Could you check a few things on this model? Use its own coordinates, in mm. A direction names the side the tool comes from. Coordinates: 2 decimals unless noted, no trailing zeros. Write each loop counter-clockwise with the first axis right and the second up, starting at its lowest first coordinate (ties: lowest second). Pieces come first, ordered by that corner, then holes.
Autodesk Inventor part; units mm, degrees
ref_plane "YZ Plane" through (0, 0, 0) normal (1, 0, 0) x (0, 1, 0)
ref_plane "XZ Plane" through (0, 0, 0) normal (0, 1, 0) x (-1, 0, 0)
ref_plane "XY Plane" through (0, 0, 0) normal (0, 0, 1) x (1, 0, 0)
sketch "Sketch1" plane through (0, 0, 0) normal (1, 0, 0) x (0, 1, 0)
  line L0 (0, 0) -> (50.8, 0)
  line L1 (50.8, 0) -> (50.8, -3.175)
  line L2 (50.8, -3.175) -> (3.175, -3.175)
  line L3 (3.175, -3.175) -> (3.175, -50.8)
  line L4 (3.175, -50.8) -> (0, -50.8)
  line L5 (0, -50.8) -> (0, 0)
  dimension "d1" = 50.8
  dimension "d2" = 3.175
  dimension "d3" = 47.625
  dimension "d4" = 47.625
  dimension "d5" = 3.175
extrude "Extrusion1" add sketch "Sketch1" along normal blind 381
sketch "Sketch2" plane through (0, 0, 0) normal (0, 0, 1) x (1, 0, 0)
  line L0 (381, 0) -> (330.2, 0)
  line L1 (0, 0) -> (381, 0)
  line L2 (330.2, 1828.8) -> (812.8, 1828.8)
  line L3 (343.6056, 50.8) -> (330.2, 0)
  line L4 (381, 0) -> (381, 50.8)
  line L5 (381, 50.8) -> (381, 0)
  line L6 (381, 50.8) -> (343.6056, 50.8)
  line L7 (0, 50.8) -> (381, 50.8)
  dimension "d9" = 50.8
  dimension "d10" = 1828.8
  dimension "d11" = 482.6
extrude "Extrusion2" cut sketch "Sketch2" against normal blind 381
properties part number "Top Frame Left"
1. Please list where these lines run through material, in increasing order: line 1 along Z through (x, y) = (194.5, 46) (3 decimals); line 2 along Y through (x, z) = (43, -18) (3 decimals).
Verdict:
line 1: z = -3.175 to 0
line 2: y = 0 to 3.175
2. I want a section at B-B on x = 312. Please give me the cut outline in (y, z) (3 decimals).
Verdict:
outline: (0, -50.8) - (3.175, -50.8) - (3.175, -3.175) - (50.8, -3.175) - (50.8, 0) - (0, 0) - close
3. I want a section at A-A on z = -9. Please give me the cut outline in (x, y) (3 decimals), plus the area to 3 significant figures.
Verdict:
outline: (0, 0) - (330.2, 0) - (331.038, 3.175) - (0, 3.175) - close
area: 1,050 mm2
4. For pin 1 (10 mm diameter, centred on x = 238, y = 20, fed in from -Z) (3 decimals); pin 2 (1 mm diameter, centred on x = 156, z = -30.5, fed in from +Y) (3 decimals), each with a flat end and sliding along its axis, tell me the tip position at first contact or that it passes through.
Verdict:
pin 1: stops at z = -3.175
pin 2: stops at y = 3.175
5. On a 3-axis mill with a long thin cutter (end or side, diameter ignored), from which of +Z, -Z, +X, -X, +Y, -Y can I reach the whole of each face in a straight line? I mean faces 1 (the face through (163, 3.175, -27)), 2 (the face through (333.955, 14.23, -2.704)). Say none if no direction works.
Verdict:
face 1: -Z, +X, -X, +Y
face 2: +Z, -Z, +X, -Y
6. I want a section at C-C on y = 46. Please give me the cut outline in (x, z) (3 decimals), plus the area to 3 significant figures.
Verdict:
outline: (0, -3.175) - (342.339, -3.175) - (342.339, 0) - (0, 0) - close
area: 1,090 mm2
